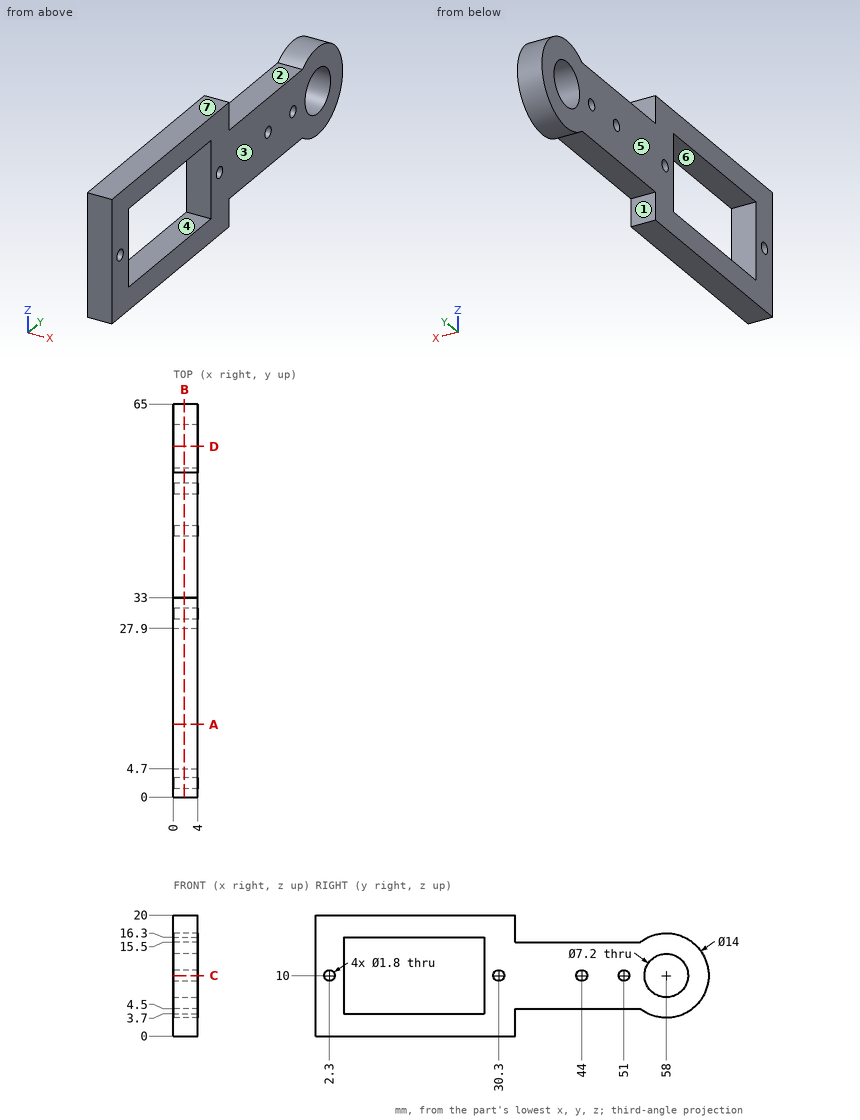
Geometry check sheet. Reference: drawing and pictorial views, mm from the part's lowest x, y, z. A direction names the side the tool comes from. Give positions to 0.01 mm unless a question says otherwise; leave off trailing zeros. Loops run counter-clockwise (first coordinate to the right, second up) from the corner with the lowest first, then second, coordinate; pieces in that order, holes last. Notation, with made-up numbers: M -9.75,-27 L 38.25,-27 A10 ccw 38.25,-23 Z; hole C 71,48 d5. An arc over 180 degrees is marked long. Use a Markdown table: item, result. Add a question column.
Q1. Sectioned sample at D-D, the plane y = 58. Record the cut outline in (x, z), then the cut area to 3 significant figures.
Q2. Mould release check, pull along Z, two halves, no side actions. Record for the marked faces 5, 6 and 7: pulls with the +Z half, pulls with the -Z half, needs draft (parallel to the pull), parting line crosses it, or undercut.
Q3. Go/stop test with flat-tipped pins: pin 1 (1 mm diameter, centred on x = 0.5, y = 44.5, fed in from +Z); pin 2 (2 mm diameter, centred on x = 1.5, z = 8.5, fed in from +Y); pin 3 (2 mm diameter, centred on x = 2, z = 1, fed in from +Y). Record where each tip stops, or that it passes through.
Q4. Sectioned sample at B-B, the plane x = 1.8. Record the cut outline in (y, z), then the cut area to 3 significant figures.
Q5. Sectioned sample at C-C, the plane z = 10. Record the cut outline in (x, y), then the cut area to 3 significant figures.
Q6. Sectioned sample at A-A, the plane y = 12. Record the cut outline in (x, z).
Q7. Tool access check on the marked faces 1, 2, 3 and 4. Record the directions out of +Z, -Z, +X, -X, +Y, -Y that give a thin tool (end or side, any length) a straight path to the whole face; none if there is none.
Q8. Scan lines: line 1 along Z through (x, y) = (0.4, 9); line 2 along Z through (x, y) = (2.15, 30.3); line 3 along Y through (x, z) = (2.5, 11). Record each from-to range of solid material in increasing order. Write a range as [from, to].
Verdict:
| question | item | result |
|---|---|---|
| 1 | outline | M 0,3 L 4,3 L 4,6.4 L 0,6.4 Z; M 0,13.6 L 4,13.6 L 4,17 L 0,17 Z |
| 1 | area | 27.2 mm^2 |
| 2 | face 5 | needs draft |
| 2 | face 6 | undercut |
| 2 | face 7 | pulls with the +Z half |
| 3 | pin 1 | z = 15.5 |
| 3 | pin 2 | y = 64.98 |
| 3 | pin 3 | y = 33 |
| 4 | outline | M 0,0 L 33,0 L 33,4.5 L 53.67,4.5 A7 ccw long 53.67,15.5 L 33,15.5 L 33,20 L 0,20 Z; hole C 2.3,10 d1.8; hole M 4.7,3.7 L 27.9,3.7 L 27.9,16.3 L 4.7,16.3 Z; hole C 30.3,10 d1.8; hole C 44,10 d1.8; hole C 51,10 d1.8; hole C 58,10 d7.2 |
| 4 | area | 678 mm^2 |
| 5 | outline | M 0,0 L 4,0 L 4,1.4 L 0,1.4 Z; M 0,3.2 L 4,3.2 L 4,4.7 L 0,4.7 Z; M 0,27.9 L 4,27.9 L 4,29.4 L 0,29.4 Z; M 0,31.2 L 4,31.2 L 4,43.1 L 0,43.1 Z; M 0,44.9 L 4,44.9 L 4,50.1 L 0,50.1 Z; M 0,51.9 L 4,51.9 L 4,54.4 L 0,54.4 Z; M 0,61.6 L 4,61.6 L 4,65 L 0,65 Z |
| 5 | area | 110 mm^2 |
| 6 | outline | M 0,0 L 4,0 L 4,3.7 L 0,3.7 Z; M 0,16.3 L 4,16.3 L 4,20 L 0,20 Z |
| 7 | face 1 | -Z, +X, -X |
| 7 | face 2 | +Z, +X, -X |
| 7 | face 3 | +Z, -Z, +X, +Y, -Y |
| 7 | face 4 | +X, -X |
| 8 | line 1 | [0, 3.7], [16.3, 20] |
| 8 | line 2 | [0, 9.1], [10.9, 20] |
| 8 | line 3 | [0, 4.7], [27.9, 54.54], [61.46, 64.93] |
